```python
from build123d import *

# Parameters (mm, degrees)
SKETCH1_R            = 1.5
BOSS_EXTRUDE1_DEPTH  = 3
FILLET5_RADIUS       = 10
FILLET5_LENGTH       = 3
FILLET2_R            = 5.4
FILLET4_R            = 5.4
SKETCH2_W            = 20.222728951
SKETCH2_H            = 4.462372077
CUT_EXTRUDE1_DEPTH   = 6
BOSS_EXTRUDE2_START  = 8
BOSS_EXTRUDE2_DEPTH  = 3
SKETCH4_W            = 16.22017041
SKETCH4_H            = 2.049534957
SKETCH4_W_2          = 13.728839959
SKETCH4_H_2          = 3.633925055
BOSS_EXTRUDE3_DEPTH  = 8
BOSS_EXTRUDE4_START  = -8
SKETCH5_R            = 1.5
BOSS_EXTRUDE4_DEPTH  = 8
SKETCH6_R            = 1.5
BOSS_EXTRUDE5_DEPTH  = 8
BOSS_EXTRUDE9_DEPTH  = 2
BOSS_EXTRUDE10_START = 2
SKETCH10_W           = 2.049534957
SKETCH10_H           = 8
BOSS_EXTRUDE10_DEPTH = 2
SKETCH11_R           = 1.5
CUT_EXTRUDE2_DEPTH   = 21


with BuildPart() as part:
    # Sketch1 → Boss-Extrude1 (new body)
    # profile 1 of 2: a face of its own
    with BuildSketch(Plane(origin=(0, 0, 0), x_dir=(1, 0, 0), z_dir=(0, 1, 0))):
        with BuildLine():
            Line((3.5, 25), (0, 25))
            Line((0, 25), (0, 15))
            Line((0, 15), (10, 0))
            Line((10, 0), (26, 0))
            Line((26, 0), (36, 15))
            Line((36, 15), (60, 15))
            Line((60, 15), (60, 25))
            Line((60, 25), (44.5, 25))
            Line((44.5, 25), (44.5, 19.6))
            Line((44.5, 19.6), (26.5, 19.6))
            Line((26.5, 19.6), (26.5, 25))
            Line((26.5, 25), (6.5, 25))
            ThreePointArc((6.5, 25), (5, 23.5), (3.5, 25))
        make_face()
        with Locations(Location((13, 5, 0), (0, 0, 270))):
            Circle(SKETCH1_R, mode=Mode.SUBTRACT)
        with Locations(Location((23, 5, 0), (0, 0, 270))):
            Circle(SKETCH1_R, mode=Mode.SUBTRACT)
    # profile 2 of 2: a face of its own
    with BuildSketch(Plane(origin=(0, 0, 0), x_dir=(1, 0, 0), z_dir=(0, 1, 0))):
        with BuildLine():
            Line((10, 45), (0, 33.819660113))
            Line((0, 33.819660113), (0, 25))
            Line((0, 25), (3.5, 25))
            ThreePointArc((3.5, 25), (5, 26.5), (6.5, 25))
            Line((6.5, 25), (26.5, 25))
            Line((26.5, 25), (26.5, 30.4))
            Line((26.5, 30.4), (44.5, 30.4))
            Line((44.5, 30.4), (44.5, 25))
            Line((44.5, 25), (60, 25))
            Line((60, 25), (60, 35))
            Line((60, 35), (36, 35))
            Line((36, 35), (26, 45))
            Line((26, 45), (10, 45))
        make_face()
    extrude(amount=BOSS_EXTRUDE1_DEPTH)

    # Fillet5: full round fillet: the end face becomes a half cylinder, R = half its width
    fillet5_face = Plane((60, 1.5, -25), x_dir=(0, -1, 0), z_dir=(1, 0, 0))  # on the end face: x along it, z out of the body
    fillet5_slab = fillet5_face.offset(-FILLET5_RADIUS / 2) * Box(FILLET5_LENGTH, 2 * FILLET5_RADIUS, FILLET5_RADIUS, mode=Mode.PRIVATE)  # the body's end, R deep
    fillet5_round = Plane((50, 1.5, -25), x_dir=(1, 0, 0), z_dir=(0, -1, 0)) * Cylinder(FILLET5_RADIUS, FILLET5_LENGTH, mode=Mode.PRIVATE)  # its axis R under the face
    add(fillet5_slab - fillet5_round, mode=Mode.SUBTRACT)

    # Fillet2
    fillet2_edges = [part.edges().sort_by_distance(p)[0] for p in [
        (26.5, 1.5, -30.4),
        (26.5, 1.5, -19.6),
    ]]
    fillet(fillet2_edges, radius=FILLET2_R - 0.0001)  # a hair under: the kernel refuses the full size

    # Fillet4
    fillet4_edges = [part.edges().sort_by_distance(p)[0] for p in [
        (44.5, 1.5, -19.6),
        (44.5, 1.5, -30.4),
    ]]
    fillet(fillet4_edges, radius=FILLET4_R - 0.0001)  # a hair under: the kernel refuses the full size

    # Sketch2 → Cut-Extrude1 (cut)
    with BuildSketch(Plane(origin=(0, 3, 0), x_dir=(1, 0, 0), z_dir=(0, 1, 0))):
        with Locations((17.936134509, 1.031658913)):
            Rectangle(SKETCH2_W, SKETCH2_H)
    extrude(amount=-CUT_EXTRUDE1_DEPTH, mode=Mode.SUBTRACT)



with BuildPart() as body_2:
    # Sketch3 → Boss-Extrude2 (new body)
    with BuildSketch(Plane(origin=(0, 3, 0), x_dir=(1, 0, 0), z_dir=(0, 1, 0)).offset(BOSS_EXTRUDE2_START)):
        Polygon((10, 45), (0, 33.819660113), (0, 15), (7.824770033, 3.262844951), (28.047498984, 3.262844951), (36, 15), (36, 35), (26, 45), align=None)
    extrude(amount=BOSS_EXTRUDE2_DEPTH)


with BuildPart() as part_1:
    add(part.part)

    add(body_2.part)  # Boss-Extrude3 merges body 2
    # Sketch4 → Boss-Extrude3 (add)
    with BuildSketch(Plane(origin=(0, 3, 0), x_dir=(1, 0, 0), z_dir=(0, 1, 0))):
        with Locations((17.889914795, 43.975232522)):
            Rectangle(SKETCH4_W, SKETCH4_H)
        with Locations((18.003368014, 5.079807479)):
            Rectangle(SKETCH4_W_2, SKETCH4_H_2)
    extrude(amount=BOSS_EXTRUDE3_DEPTH)

    # Sketch5 → Boss-Extrude4 (add)
    with BuildSketch(Plane(origin=(0, 14, 0), x_dir=(1, 0, 0), z_dir=(0, 1, 0)).offset(BOSS_EXTRUDE4_START)):
        with Locations(Location((5, 25, 0), (0, 0, 270))):
            Circle(SKETCH5_R)
    extrude(amount=BOSS_EXTRUDE4_DEPTH)

    # Sketch6 → Boss-Extrude5 (add)
    with BuildSketch(Plane(origin=(0, 14, 0), x_dir=(1, 0, 0), z_dir=(0, 1, 0))):
        with Locations(Location((31.9, 25, 0), (0, 0, 270))):
            Circle(SKETCH6_R)
    extrude(amount=-BOSS_EXTRUDE5_DEPTH)

    # Sketch7 → Boss-Extrude9 (add)
    # profile 1 of 2: a face of its own
    with BuildSketch(Plane.ZY.offset(-9.77982959)):
        with BuildLine():
            ThreePointArc((-42.829650223, 14), (-72.227622353, 7), (-42.829650223, 0))
            Line((-42.829650223, 0), (-42.829650223, 14))
        make_face()
        Polygon((-44.753841998, 3), (-45, 3), (-45, 11), (-44.753841998, 11), (-42.950465043, 11), (-42.950465043, 3), align=None, mode=Mode.SUBTRACT)
    # profile 2 of 2: a face of its own
    with BuildSketch(Plane.ZY.offset(-9.77982959)):
        Polygon((-45, 11), (-45, 3), (-44.753841998, 3), (-42.950465043, 3), (-42.950465043, 11), (-44.753841998, 11), align=None)
    extrude(amount=BOSS_EXTRUDE9_DEPTH)

    # Sketch10 → Boss-Extrude10 (add)
    # profile 1 of 2: a face of its own
    with BuildSketch(Plane(origin=(26, 0, 0), x_dir=(0, 0, -1), z_dir=(1, 0, 0)).offset(BOSS_EXTRUDE10_START)):
        with BuildLine():
            ThreePointArc((72.227622353, 7), (60.293097644, 22.109936841), (42.829650223, 14))
            Line((42.829650223, 14), (42.829650223, 0))
            ThreePointArc((42.829650223, 0), (60.293097644, -8.109936841), (72.227622353, 7))
        make_face()
        with Locations((43.975232522, 7)):
            Rectangle(SKETCH10_W, SKETCH10_H, mode=Mode.SUBTRACT)
    # profile 2 of 2: a face of its own
    with BuildSketch(Plane(origin=(26, 0, 0), x_dir=(0, 0, -1), z_dir=(1, 0, 0)).offset(BOSS_EXTRUDE10_START)):
        with Locations((43.975232522, 7)):
            Rectangle(SKETCH10_W, SKETCH10_H)
    extrude(amount=-BOSS_EXTRUDE10_DEPTH)

    # Sketch11 → Cut-Extrude2 (cut)
    with BuildSketch(Plane.ZY.offset(-7.77982959)):
        with Locations((-56.695245471, 7)):
            Circle(SKETCH11_R)
    extrude(amount=-CUT_EXTRUDE2_DEPTH, mode=Mode.SUBTRACT)


solid = part_1.part
```
Check sheet for the modelled part. Datum: model origin and axes. Units: mm. A direction names the side the tool comes from. Give positions to 0.01 mm unless a question says otherwise; leave off trailing zeros. Write each loop counter-clockwise with the first axis right and the second up, starting at its lowest first coordinate (ties: lowest second). Pieces come first, ordered by that corner, then holes.
Item 1: Cross-section at A-A (z = -8). Enter the section's corners in (x, y).
Item 2: Draft check along Y on faces 1 (the face through (9, 7, -42.83)), 2 (the face through (32, 1, -9)), 3 (the face through (23, 0, -24)). Enter one of: released by +Y, released by -Y, zero draft, split by the parting line, or undercut.
Item 3: Cross-section at C-C (z = -28.5). Enter the section's corners in (x, y), and give its area (3 significant figures).
Item 4: Scan lines: L1, parallel to X at y = 2.35, z = -25; L2, parallel to X at y = -5, z = -52; L3, parallel to X at y = 2, z = -5. Record each from-to range of solid material in increasing order.
Item 5: Access from +Z, -Z, +X, -X, +Y, -Y to the whole of each face (thin tool, end or side, straight path). Record for faces 4 (the face through (42.876, 1.521, -28.86)), 5 (the face through (18, 7, -3.263)), 6 (the face through (36, 12, -25)), 7 (the face through (28.04, 1.521, -28.776)), 8 (the face through (18, 7, -6.897)).
Item 6: Gauge pin test, flat ends, axial feed: pin 1 (3.5 mm diameter, centred on x = 34, y = 2, fed in from +Z) (3 decimals); pin 2 (0.9 mm diameter, centred on x = 43.5, y = 1.5, fed in from +Z); pin 3 (4 mm diameter, centred on x = 13, z = -5, fed in from +Y); pin 4 (12 mm diameter, centred on x = 45, y = 14.5, fed in from -Z). Record the tip position at first contact, or that the pin passes through.
Item 7: Cross-section at D-D (y = 17). Enter the section's corners in (x, z), and give its area (3 significant figures).
Item 8: Cross-section at B-B (x = 13). Enter the section's corners in (y, z).
Report:
1. outline: (4.67, 0) - (31.33, 0) - (31.33, 3) - (4.67, 3) - close; (4.67, 11) - (31.26, 11) - (31.26, 14) - (4.67, 14) - close
2. face 1: undercut
2. face 2: zero draft
2. face 3: released by -Y
3. outline: (0, 0) - (27.79, 0) - (27.79, 3) - (0, 3) - close; (0, 11) - (36, 11) - (36, 14) - (0, 14) - close; (43.21, 0) - (59.37, 0) - (59.37, 3) - (43.21, 3) - close
3. area: 240 mm2
4. L1: x = 0 to 3.5, 6.5 to 26.5, 44.5 to 60
4. L2: x = 7.78 to 9.78, 26 to 28
4. L3: x = 6.67 to 11.5, 14.5 to 21.5, 24.5 to 29.33
5. face 4: +Y, -Y
5. face 5: +Z, -X, +Y, -Y
5. face 6: +Z, -Z, +X, +Y
5. face 7: -Y
5. face 8: +X, -X
6. pin 1: stops at z = -9.375
6. pin 2: stops at z = -15
6. pin 3: stops at y = 14
6. pin 4: passes through
7. outline: (7.78, -68.58) - (9.78, -68.58) - (9.78, -44.81) - (7.78, -44.81) - close; (26, -68.58) - (28, -68.58) - (28, -44.81) - (26, -44.81) - close
7. area: 95.1 mm2
8. outline: (0, -45) - (14, -45) - (14, -3.26) - (0, -3.26) - (0, -3.5) - (3, -3.5) - (3, -6.5) - (0, -6.5) - close; hole (3, -42.95) - (11, -42.95) - (11, -6.9) - (3, -6.9) - close
